Here's how the part is built. I have some questions about the finished solid (model axes, mm). A direction names the side the tool comes from. Give positions to 0.01 mm unless a question says otherwise; leave off trailing zeros. Write each loop counter-clockwise with the first axis right and the second up, starting at its lowest first coordinate (ties: lowest second). Pieces come first, ordered by that corner, then holes. Notation, with made-up numbers: (39.5, 62.5) - (87.5, 62.5) arc R15 ccw to (87.5, 90.5) - close; hole circle Ø11 at (15.25, 66.5). An arc over 180 degrees is marked (long way). Use a Markdown table: item, result.
```python
from build123d import *

# Parameters (mm, degrees)
BOSS_EXTRUDE1_DEPTH     = 20
CUT_EXTRUDE1_DEPTH      = 286.306420625
CUT_EXTRUDE1_DEPTH_BACK = 286.306420625
SKETCH3_W               = 16
SKETCH3_H               = 16.536122988


with BuildPart() as part:
    # Sketch1 → Boss-Extrude1 (new body)
    with BuildSketch(Plane.XY):
        Polygon((-48.421052632, 24.605263158), (271.988947368, 24.605263158), (283.538947368, 4.605263158), (-59.971052632, 4.605263158), align=None)
    extrude(amount=BOSS_EXTRUDE1_DEPTH)

    # Sketch3 → Cut-Extrude1 (cut, two sides: drawn at the far end of the back side and taken through both)
    with BuildSketch(Plane(origin=(0, 0, 0), x_dir=(0, 0, -1), z_dir=(1, 0, 0)).offset(-CUT_EXTRUDE1_DEPTH_BACK)):
        with Locations((-10, 14.605263158)):
            Rectangle(SKETCH3_W, SKETCH3_H)
    extrude(amount=CUT_EXTRUDE1_DEPTH + CUT_EXTRUDE1_DEPTH_BACK, mode=Mode.SUBTRACT)


solid = part.part
```
Item 1: If we section it at A-A, the plane x = -12: Write out the boundary of the cut face in (y, z).
Values:
| item | result |
|---|---|
| outline | (4.61, 0) - (24.61, 0) - (24.61, 20) - (4.61, 20) - close; hole (6.34, 2) - (22.87, 2) - (22.87, 18) - (6.34, 18) - close |
Item 2: Thinking about a two-plate mould opening in Y: for faces 3 (the flat face through (114, 15, 20)), 4 (the flat face through (109, 14, 2)), 5 (the flat face through (-54.277, 14.465, 18.749)), which applies, +Y half, -Y half, draft (parallel to the pull), parting line (faces both ways), or undercut?
Values:
| item | result |
|---|---|
| face 3 | draft |
| face 4 | undercut |
| face 5 | +Y half |
Item 3: Will these pins go through, and if not, where does the flat tip stop? pin 1 Ø6 at (x, y) = (96, 18) entering from -Z; pin 2 Ø12 at (y, z) = (12.5, 15) entering from +X; pin 3 Ø1.5 at (y, z) = (22.5, 10) entering from -X.
Values:
| item | result |
|---|---|
| pin 1 | stops at z = 0 |
| pin 2 | stops at x = 281.98 |
| pin 3 | stops at x = -49.42 |
Item 4: If we section it at B-B, the plane y = 16.5: Write out the boundary of the cut face in (x, z).
Values:
| item | result |
|---|---|
| outline | (-53.1, 0) - (276.67, 0) - (276.67, 2) - (-53.1, 2) - close; (-53.1, 18) - (276.67, 18) - (276.67, 20) - (-53.1, 20) - close |
Item 5: If we section it at C-C, the plane z = 14.75: Write out the boundary of the cut face in (x, y).
Values:
| item | result |
|---|---|
| outline | (-59.97, 4.61) - (283.54, 4.61) - (282.54, 6.34) - (-58.97, 6.34) - close; (-49.42, 22.87) - (272.99, 22.87) - (271.99, 24.61) - (-48.42, 24.61) - close |
Item 6: For faces 1 (the flat face through (109, 14, 18)), 2 (the flat face through (114, 15, 0)), which set-ups out of +Z, -Z, +X, -X, +Y, -Y let a thin tool reach every point of the face, with its end or its side?
Values:
| item | result |
|---|---|
| face 1 | +X, -X |
| face 2 | -Z, +X, -X, +Y, -Y |
Item 7: I need wall thicknesses on line 1 along Y through (x, z) = (173.5, 6); line 2 along Z through (x, y) = (203, 8); line 3 along X through (y, z) = (11.5, 19). Which ranges of each line are inside material? Lowest first, please. Write a range as [from, to].
Values:
| item | result |
|---|---|
| line 1 | y = [4.61, 6.34], [22.87, 24.61] |
| line 2 | z = [0, 2], [18, 20] |
| line 3 | x = [-55.99, 279.56] |
